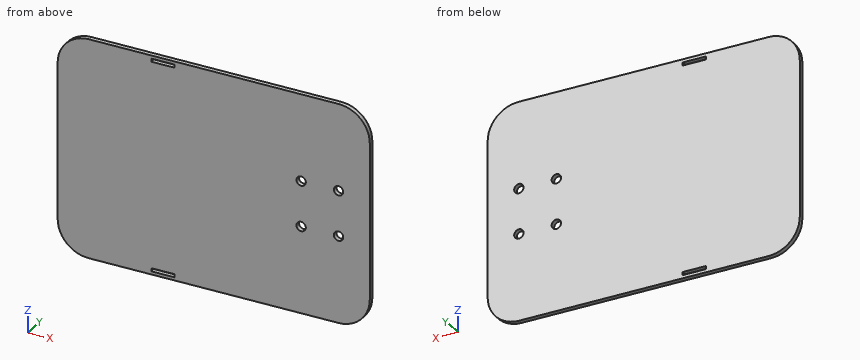
Autodesk Inventor part; units mm, degrees
ref_plane "YZ Plane" through (0, 0, 0) normal (1, 0, 0) x (0, 1, 0)
ref_plane "XZ Plane" through (0, 0, 0) normal (0, 1, 0) x (-1, 0, 0)
ref_plane "XY Plane" through (0, 0, 0) normal (0, 0, 1) x (1, 0, 0)
sketch "Szkic1" plane through (0, 0, 0) normal (0, 1, 0) x (-1, 0, 0)
  line L0 (0, 0) -> (-200, 0)
  line L1 (-200, 0) -> (-200, 140)
  line L2 (-200, 140) -> (0, 140)
  line L3 (0, 140) -> (0, 0)
  dimension "d0" = 200
  dimension "d1" = 140
extrude "Wyciągnięcie proste1" add sketch "Szkic1" along normal blind 3
sketch "Szkic2" plane through (0, 3, 0) normal (0, 1, 0) x (1, 0, 0)
  line L0 (0, 0) -> (50, 0)
  line L1 (200, 0) -> (0, 0)
  line L2 (50, 0) -> (60, 0)
  line L3 (60, 0) -> (60, -2)
  line L4 (60, -2) -> (75, -2)
  line L5 (75, -2) -> (75, -4)
  line L6 (75, -4) -> (60, -4)
  line L7 (60, -4) -> (60, -2)
  line L8 (0, 0) -> (0, -140)
  line L9 (0, -70) -> (200, -70)
  line L10 (200, -140) -> (200, 0)
  line L11 (60, -140) -> (60, -138)
  line L12 (60, -138) -> (75, -138)
  line L13 (75, -138) -> (75, -136)
  line L14 (75, -136) -> (60, -136)
  line L15 (60, -136) -> (60, -138)
  dimension "d4" = 50
  dimension "d5" = 10
  dimension "d6" = 2
  dimension "d7" = 15
  dimension "d8" = 2
extrude "Wyciągnięcie proste2" cut sketch "Szkic2" against normal blind 3 contours L4 L5 L6 L7 | L15 L14 L13 L12
sketch "Szkic3" plane through (0, 3, 0) normal (0, 1, 0) x (1, 0, 0)
  line L0 (200, -140) -> (200, 0)
  line L1 (0, -140) -> (200, -140)
  line L2 (200, 0) -> (180, 0)
  line L3 (180, 0) -> (180, -140)
  line L4 (180, -140) -> (200, -140)
  line L5 (200, -140) -> (200, 0)
  line L6 (180, -70) -> (180, -53)
  line L7 (180, -53) -> (180, -55.5)
  circle A0 centre (180, -55.5) radius 3
  line L8 (180, -55.5) -> (156, -55.5)
  circle A1 centre (156, -55.5) radius 3
  line L9 (200, -70) -> (129.0719, -70)
  circle A2 centre (180, -84.5) radius 3
  circle A3 centre (156, -84.5) radius 3
  point P0 (0, 0)
  dimension "d11" = 20
  dimension "d12" = 17
  dimension "d13" = 2.5
  dimension "d14" = 6
  dimension "d15" = 24
  dimension "d16" = 6
extrude "Wyciągnięcie proste3" cut sketch "Szkic3" against normal blind 3 contours A1 | A2 L3 | L3 A2 | A0 L8 L3 | L3 A0 | L3 L8 A0 | A3
fillet "Zaokrąglenie1" radius 20 4 edges at (0, 1.5, 140) (0, 1.5, 0) (200, 1.5, 0) (200, 1.5, 140)
properties part number "podstawa"
Can you work these out from the model? Positions are in its coordinate system, mm. Round coordinates to 2 decimals unless told otherwise and drop trailing zeros. Loops run counter-clockwise (first coordinate to the right, second up) from the corner with the lowest first, then second, coordinate; pieces in that order, holes last. Notation, with made-up numbers: (-34, 32) - (-2, 32) arc R26 ccw to (-2, 52) - close; hole circle Ø5 at (40, 62.25). An arc over 180 degrees is marked (long way). Write item = value, one per line. Start each with the question number.
(1) If we section it at C-C (y = 0.8): Please give me the cut outline in (x, z).
(2) If we section it at A-A (x = 156): Please give me the cut outline in (y, z).
(3) If we section it at B-B (z = 84.5): Please give me the cut outline in (x, y).
(4) If I drill on probe 1 along X at (y, z) = (1.4, 84.5); probe 2 along Z at (x, y) = (156, 2.3); probe 3 along X at (y, z) = (2.5, 121), over which ranges is the centre line in solid material (lowest first)? Write a range as [from, to].
(5) For P1, Ø0.6, axis at y = 1, z = 136.5, coming from the +X side; P2, Ø12, axis at x = 147, z = 77.5, coming from the -Y side; P3, Ø1, axis at y = 1, z = 3, coming from the +X side, each with a flat end and sliding along its axis, tell me the tip position at first contact or that it passes through.
Ans:
q1.outline = (0, 20) arc R20 ccw to (20, 0) - (180, 0) arc R20 ccw to (200, 20) - (200, 120) arc R20 ccw to (180, 140) - (20, 140) arc R20 ccw to (0, 120) - close; hole (60, 2) - (75, 2) - (75, 4) - (60, 4) - close; hole (60, 136) - (75, 136) - (75, 138) - (60, 138) - close; hole circle Ø6 at (156, 55.5); hole circle Ø6 at (156, 84.5); hole circle Ø6 at (180, 55.5); hole circle Ø6 at (180, 84.5)
q2.outline = (0, 0) - (3, 0) - (3, 52.5) - (0, 52.5) - close; (0, 58.5) - (3, 58.5) - (3, 81.5) - (0, 81.5) - close; (0, 87.5) - (3, 87.5) - (3, 140) - (0, 140) - close
q3.outline = (0, 0) - (153, 0) - (153, 3) - (0, 3) - close; (159, 0) - (177, 0) - (177, 3) - (159, 3) - close; (183, 0) - (200, 0) - (200, 3) - (183, 3) - close
q4.probe_1 = [0, 153], [159, 177], [183, 200]
q4.probe_2 = [0, 52.5], [58.5, 81.5], [87.5, 140]
q4.probe_3 = [0.03, 199.97]
q5.P1 = 191.73
q5.P2 = 0
q5.P3 = 191.3
